Could you check a few things on this model? Use its own coordinates, in mm. Face numbers are marked on the shaded views. A direction names the side the tool comes from. Coordinates: 2 decimals unless noted, no trailing zeros. Loops run counter-clockwise (first coordinate to the right, second up) from the corner with the lowest first, then second, coordinate; pieces in that order, holes last. Notation, with made-up numbers: (63, -36) -> (104, -36) arc R21 cw to (104, -21) -> close; hole circle Ø1 at (11, -17.5). An arc over 180 degrees is marked (long way). One line per question, with ' | ' between items.
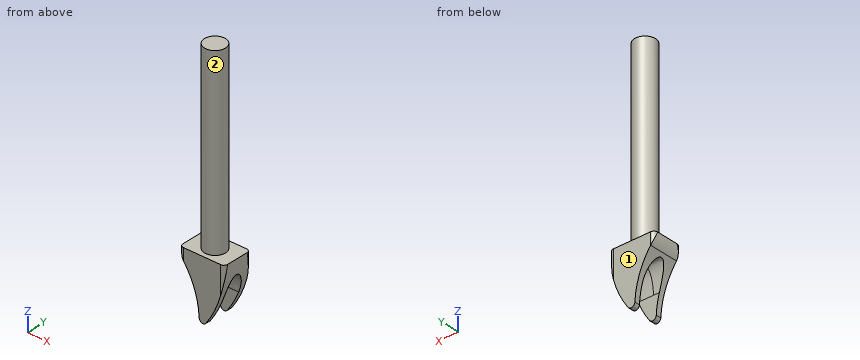
from build123d import *

# Parameters (mm, degrees)
F0_R     = 14
F1_DEPTH = 244
F2_W     = 60
F2_H     = 40
F3_DEPTH = 80
F4_R     = 5
F6_DEPTH = 40
F8_DEPTH = 35


with BuildPart() as f1:
    # F0 (on Top) → F1 (new body)
    with BuildSketch(Plane.XY):
        Circle(F0_R)
    extrude(amount=F1_DEPTH)

    # F2 (on Top) → F3 (join)
    with BuildSketch(Plane.XY):
        Rectangle(F2_W, F2_H)
    extrude(amount=-F3_DEPTH)

    # F4
    f4_edges = [f1.edges().sort_by_distance(p)[0] for p in [
        (30, -20, -40),
        (-30, -20, -40),
        (30, 20, -40),
        (-30, 20, -40),
    ]]
    fillet(f4_edges, radius=F4_R)

    # F5 (on Front) → F6 (cut, symmetric)
    with BuildSketch(Plane.XZ):
        with BuildLine():
            Line((-30, 0), (-30, -85))
            Line((-30, -85), (30, -85))
            Line((30, -85), (30, 0))
            ThreePointArc((30, 0), (23.6684739344, -40.85858313), (5.2677953275, -77.8846153846))
            ThreePointArc((5.2677953275, -77.8846153846), (-0.2236501523, -79.7978199094), (-3.8113000271, -75.2212389381))
            ThreePointArc((-3.8113000271, -75.2212389381), (-9.8768127885, -44.0150908016), (-24.7651593513, -15.9268145426))
            ThreePointArc((-24.7651593513, -15.9268145426), (-28.6577337776, -8.3825261421), (-30, 0))
        make_face()
    extrude(amount=F6_DEPTH, both=True, mode=Mode.SUBTRACT)

    # F7 (on Right) → F8 (cut, symmetric)
    with BuildSketch(Plane.YZ):
        with BuildLine():
            Line((13, -80), (13, -50))
            add(Edge.make_bspline(
                [(13, -50), (13, -20), (0, -20), (-13, -20), (-13, -50)],
                knots=[1.5707963268, 1.5707963268, 1.5707963268, 3.1415926536, 3.1415926536, 4.7123889804, 4.7123889804, 4.7123889804], degree=2, weights=[1, 0.7071067812, 1, 0.7071067812, 1]))
            Line((-13, -50), (-13, -80))
            Line((-13, -80), (13, -80))
        make_face()
    extrude(amount=F8_DEPTH, both=True, mode=Mode.SUBTRACT)


solid = f1.part
1) If we section it at A-A on z = -58: Please give me the cut outline in (x, y).
Data:
outline: (-5.97, -20) -> (16.91, -20) -> (16.91, -13) -> (-5.97, -13) -> close; (-5.97, 13) -> (16.91, 13) -> (16.91, 20) -> (-5.97, 20) -> close
2) On a 3-axis mill with a long thin cutter (end or side, diameter ignored), from which of +Z, -Z, +X, -X, +Y, -Y can I reach the whole of each face in a straight line? I mean the marked faces 1 and 2. Say none if no direction works.
Data:
face 1: +Z, -Z, +X, -X, +Y | face 2: +Z
3) If we section it at B-B on z = 114: Please give me the cut outline in (x, y), and give its area (3 significant figures).
Data:
outline: circle Ø28 at (0, 0) | area: 616 mm²
4) I'm going to push flat-ended pins straight in: pin 1 Ø1.5 at (y, z) = (6.5, 41) entering from -X; pin 2 Ø12 at (x, y) = (18.5, 8) entering from +Z; pin 3 Ø3 at (y, z) = (10.5, 104.5) entering from +X. Where does each tip first touch, or does it pass through?
Data:
pin 1: x = -12.76 | pin 2: z = 0 | pin 3: x = 10.72
5) I need wall thicknesses on line 1 along Y through (x, z) = (-1.5, -56.5); line 2 along Y through (x, z) = (-1, 35); line 3 along Y through (x, z) = (-12, -27). Which ranges of each line are inside material? Lowest first, please. Write a range as from..to.
Data:
line 1: -20..-13, 13..20 | line 2: -13.96..13.96 | line 3: -20..-8.35, 8.35..20
